Here's how the part is built. I have some questions about the finished solid (model axes, mm). Face numbers are marked on the shaded views. A direction names the side the tool comes from. Round coordinates to 2 decimals unless told otherwise and drop trailing zeros. Order: outer loops, then holes, each group sorted by start corner. A loop starts at its lowest first (then second) coordinate and runs counter-clockwise, first axis right, second up. Notation, with made-up numbers: (73, 68.5) - (110, 68.5) arc R18 cw to (110, 74.5) - close; hole circle Ø1 at (42, 5.25). An arc over 180 degrees is marked (long way). One line per item, written item: value.
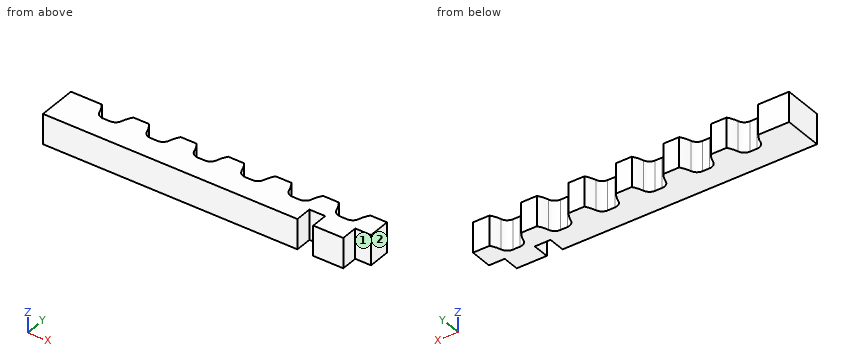
from build123d import *

# Parameters (mm, degrees)
CROQUIS4_W              = 40
CROQUIS4_H              = 4.9
SALIENTE_EXTRUIR1_DEPTH = 3.8
CORTAR_EXTRUIR1_DEPTH   = 5
REDONDEO1_R             = 1
MATRIZL1_COUNT          = 6
MATRIZL1_PITCH          = 6
REDONDEO1_OF_MATRIZL1_R = 1
CROQUIS7_W              = 2
CROQUIS7_H              = 4.2
CORTAR_EXTRUIR2_DEPTH   = 10


with BuildPart() as part:
    # Croquis4 → Saliente-Extruir1 (new body)
    with BuildSketch(Plane.XY):
        Rectangle(CROQUIS4_W, CROQUIS4_H)
    extrude(amount=SALIENTE_EXTRUIR1_DEPTH)

    # Croquis5 → Cortar-Extruir1 (cut)
    with BuildSketch(Plane.XY.offset(3.8)):
        with BuildLine():
            Line((-16.122428878, 2.488752454), (-12.062122986, 2.488752454))
            ThreePointArc((-12.062122986, 2.488752454), (-12.575562017, 1.545062529), (-12.814503922, 0.497648057))
            Line((-12.814503922, 0.497648057), (-15.370047942, 0.497648057))
            ThreePointArc((-15.370047942, 0.497648057), (-15.608989847, 1.545062529), (-16.122428878, 2.488752454))
        make_face()
    cortar_extruir1 = extrude(amount=-CORTAR_EXTRUIR1_DEPTH, mode=Mode.SUBTRACT)

    # Redondeo1
    redondeo1_edges = [part.edges().sort_by_distance(p)[0] for p in [
        (-12.814503922, 0.497648057, 1.9),
        (-15.370047942, 0.497648057, 1.9),
    ]]
    fillet(redondeo1_edges, radius=REDONDEO1_R)

    # MatrizL1: Cortar-Extruir1 ×6
    with Locations(*[(i * MATRIZL1_PITCH, 0, 0) for i in range(1, MATRIZL1_COUNT)]):
        add(cortar_extruir1, mode=Mode.SUBTRACT)

    # Redondeo1 of MatrizL1
    redondeo1_of_matrizl1_edges = [part.edges().sort_by_distance(p)[0] for p in [
        (-6.814503922, 0.497648057, 1.9),
        (-9.370047942, 0.497648057, 1.9),
        (-0.814503922, 0.497648057, 1.9),
        (-3.370047942, 0.497648057, 1.9),
        (5.185496078, 0.497648057, 1.9),
        (2.629952058, 0.497648057, 1.9),
        (11.185496078, 0.497648057, 1.9),
        (8.629952058, 0.497648057, 1.9),
        (17.185496078, 0.497648057, 1.9),
        (14.629952058, 0.497648057, 1.9),
    ]]
    fillet(redondeo1_of_matrizl1_edges, radius=REDONDEO1_OF_MATRIZL1_R)

    # Croquis7 → Cortar-Extruir2 (cut)
    with BuildSketch(Plane.XY.offset(3.8)):
        with Locations((19, -2.45)):
            Rectangle(CROQUIS7_W, CROQUIS7_H)
        with Locations((13.2, -2.45)):
            Rectangle(CROQUIS7_W, CROQUIS7_H)
    extrude(amount=-CORTAR_EXTRUIR2_DEPTH, mode=Mode.SUBTRACT)


solid = part.part
Q1. If we section it at A-A, the plane y = -1.4: Please give me the cut outline in (x, z).
Results list:
outline: (-20, 0) - (12.2, 0) - (12.2, 3.8) - (-20, 3.8) - close; (14.2, 0) - (18, 0) - (18, 3.8) - (14.2, 3.8) - close
Q2. Which directions (+Z, -Z, +X, -X, +Y, -Y) give clear straight access to the entire face, cutting with the end or side of a thin tool? Please do the marked faces 1 and 2.
Results list:
face 1: +Z, -Z, +X, -Y
face 2: +Z, -Z, +X, +Y, -Y
Q3. If we section it at C-C, the plane x = -14: Please give me the cut outline in (y, z), then the cut area to 3 significant figures.
Results list:
outline: (-2.45, 0) - (0.5, 0) - (0.5, 3.8) - (-2.45, 3.8) - close
area: 11.2 mm²
Q4. If we section it at B-B, the plane y = 1.65: Please give me the cut outline in (x, z).
Results list:
outline: (-20, 0) - (-15.65, 0) - (-15.65, 3.8) - (-20, 3.8) - close; (-12.53, 0) - (-9.65, 0) - (-9.65, 3.8) - (-12.53, 3.8) - close; (-6.53, 0) - (-3.65, 0) - (-3.65, 3.8) - (-6.53, 3.8) - close; (-0.53, 0) - (2.35, 0) - (2.35, 3.8) - (-0.53, 3.8) - close; (5.47, 0) - (8.35, 0) - (8.35, 3.8) - (5.47, 3.8) - close; (11.47, 0) - (14.35, 0) - (14.35, 3.8) - (11.47, 3.8) - close; (17.47, 0) - (20, 0) - (20, 3.8) - (17.47, 3.8) - close
Q5. Will these pins go through, and if not, where does the flat tip stop? pin 1 (1 mm diameter, centred on x = 13, z = 3, fed in from -Y); pin 2 (1 mm diameter, centred on x = 10, z = 2.5, fed in from +Y); pin 3 (1.7 mm diameter, centred on y = -2, z = 1.5, fed in from +X).
Results list:
pin 1: y = -0.35
pin 2: y = 0.51
pin 3: x = 18
Q6. If I drill on line 1 along X through (y, z) = (-1.65, 0.7); line 2 along Y through (x, z) = (15.5, 3.65); line 3 along Y through (x, z) = (13.5, 0.45), over which ranges is the centre line in solid material (lowest first)?
Results list:
line 1: -20 to 12.2, 14.2 to 18
line 2: -2.45 to 0.5
line 3: -0.35 to 2.45
